The listing builds one solid part. Answer for the finished solid, in the listing's coordinates (mm). A direction names the side the tool comes from. Round coordinates to 2 decimals unless told otherwise and drop trailing zeros. Write each loop counter-clockwise with the first axis right and the second up, starting at its lowest first coordinate (ties: lowest second). Pieces come first, ordered by that corner, then holes. Notation, with made-up numbers: (-22, 45.25) - (30, 45.25) arc R19 ccw to (30, 82.25) - close; hole circle Ø6 at (16.5, -38). An arc over 180 degrees is marked (long way). Answer in a Markdown table with one row per item.
from build123d import *

# Parameters (mm, degrees)
BOSS_EXTRUDE1_DEPTH       = 419.1
F_8_CLEARANCE_HOLE1_D     = 4.9149
F_8_CLEARANCE_HOLE1_DEPTH = 9.652
F_8_CLEARANCE_HOLE1_TIP   = 1.476584928


with BuildPart() as part:
    # Sketch1 → Boss-Extrude1 (new body)
    with BuildSketch(Plane(origin=(0, 0, 0), x_dir=(1, 0, 0), z_dir=(0, 1, 0))):
        Polygon((-17.170187141, 1.020273681), (382.879812859, 1.020273681), (382.879812859, -8.504726319), (408.279812859, -8.504726319), (408.279812859, -18.029726319), (382.879812859, -18.029726319), (-17.170187141, -18.029726319), (-42.570187141, -18.029726319), (-42.570187141, -8.504726319), (-17.170187141, -8.504726319), align=None)
    extrude(amount=BOSS_EXTRUDE1_DEPTH)

    # #8 Clearance Hole1
    with Locations(Plane.XY.offset(18.029726319)):
        with Locations((-29.870187141, 393.7), (-29.870187141, 320.04), (-29.870187141, 246.38), (-29.870187141, 172.72), (-29.870187141, 99.06), (-29.870187141, 25.4), (395.579812859, 25.4), (395.579812859, 99.06), (395.579812859, 172.72), (395.579812859, 246.38), (395.579812859, 320.04), (395.579812859, 393.7)):
            Hole(F_8_CLEARANCE_HOLE1_D / 2, depth=F_8_CLEARANCE_HOLE1_DEPTH)
            with Locations((0, 0, -(F_8_CLEARANCE_HOLE1_DEPTH + F_8_CLEARANCE_HOLE1_TIP / 2))):  # 118° drill point
                Cone(0, F_8_CLEARANCE_HOLE1_D / 2, F_8_CLEARANCE_HOLE1_TIP, mode=Mode.SUBTRACT)


solid = part.part
(1) For faces 1 (the flat face through (-17.17, 207, 4)), 2 (the flat face through (395, 207, 8.505)), 3 (the flat face through (180, 207, -1.02)), determine the directions among +Z, -Z, +X, -X, +Y, -Y from which every point of the face is accessible in a straight line to the end or side of a thin tool.
Checked values:
| item | result |
|---|---|
| face 1 | -Z, -X, +Y, -Y |
| face 2 | -Z, +X, +Y, -Y |
| face 3 | -Z, +X, -X, +Y, -Y |
(2) Section B-B (z = 5.25) is taken. Give the vertices of the cut face in (x, y), and give its area (3 significant figures).
Checked values:
| item | result |
|---|---|
| outline | (-17.17, 0) - (382.88, 0) - (382.88, 419.1) - (-17.17, 419.1) - close |
| area | 168,000 mm2 |
(3) Find the intervals of material crossed by line 1 (X direction, y = 246.38, z = 13); line 2 (X direction, y = 394.5, z = 16.75); line 3 (X direction, y = 266, z = 7.5), in increasing order.
Checked values:
| item | result |
|---|---|
| line 1 | x = -42.57 to -32.33, -27.41 to 393.12, 398.04 to 408.28 |
| line 2 | x = -42.57 to -32.19, -27.55 to 393.26, 397.9 to 408.28 |
| line 3 | x = -17.17 to 382.88 |
(4) Section A-A (y = 124.5) is taken. Give the vertices of the cut face in (x, z), and give its area (3 significant figures).
Checked values:
| item | result |
|---|---|
| outline | (-42.57, 8.5) - (-17.17, 8.5) - (-17.17, -1.02) - (382.88, -1.02) - (382.88, 8.5) - (408.28, 8.5) - (408.28, 18.03) - (-42.57, 18.03) - close |
| area | 8,100 mm2 |
(5) Flat-ended cylindrical pins translate along their axes: pin 1 (7.5 mm diameter, centred on x = 398, y = 114.5, fed in from -Z); pin 2 (3 mm diameter, centred on x = 143, z = 10, fed in from -Y); pin 3 (10 mm diameter, centred on y = 228, z = 1.5, fed in from +X). Find the tip coordinate at first contact, or state that the pin passes through.
Checked values:
| item | result |
|---|---|
| pin 1 | stops at z = 8.5 |
| pin 2 | stops at y = 0 |
| pin 3 | stops at x = 382.88 |
